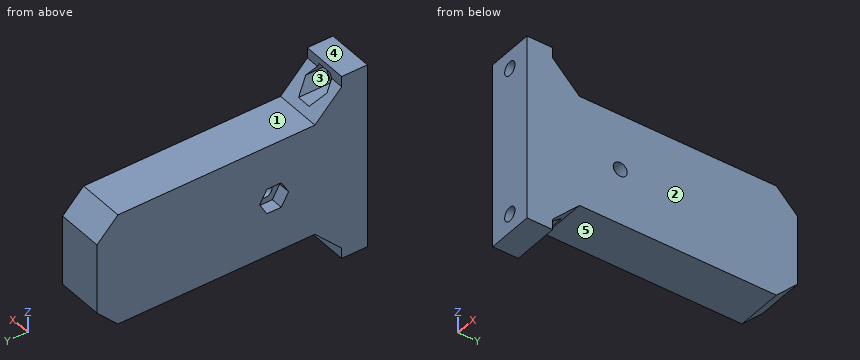
Autodesk Inventor part; units mm, degrees
ref_plane "YZ Plane" through (0, 0, 0) normal (1, 0, 0) x (0, 1, 0)
ref_plane "XZ Plane" through (0, 0, 0) normal (0, 1, 0) x (-1, 0, 0)
ref_plane "XY Plane" through (0, 0, 0) normal (0, 0, 1) x (1, 0, 0)
sketch "Эскиз1" plane through (0, 0, 0) normal (0, 1, 0) x (-1, 0, 0)
  line L0 (-5, 20) -> (5, 20)
  line L1 (5, 20) -> (5, -20)
  line L2 (5, -20) -> (-5, -20)
  line L3 (-5, -20) -> (-5, 20)
  line L4 (-5, 20) -> (5, -20) construction
  line L5 (5, 20) -> (-5, -20) construction
  point P0 (0, 0)
  dimension "d0" = 10
  dimension "d1" = 40
extrude "Выдавливание1" add sketch "Эскиз1" along normal blind 3
sketch "Эскиз2" plane through (0, 3, 0) normal (0, 1, 0) x (1, 0, 0)
  line L0 (-5, 20) -> (-5, -20)
  line L1 (5, -12) -> (-5, -12)
  line L2 (-5, -12) -> (-5, 12)
  line L3 (-5, 12) -> (5, 12)
  line L4 (5, 12) -> (5, -12)
  line L5 (5, -12) -> (-5, 12) construction
  line L6 (-5, -12) -> (5, 12) construction
  point P0 (0, 0)
  dimension "d4" = 24
extrude "Выдавливание2" add sketch "Эскиз2" along normal blind 55
sketch "Эскиз3" plane through (0, 3, 0) normal (0, 1, 0) x (1, 0, 0)
  circle A0 centre (0, -16) radius 1.5
  line L0 (-5, -12) -> (-5, -20)
  line L1 (-5, -20) -> (5, -20)
  point P0 (0, 0)
  dimension "d7" = 3
  dimension "d8" = 5
  dimension "d9" = 4
extrude "Выдавливание3" cut sketch "Эскиз3" against normal blind 20
mirror "Зеркальное отражение1" about plane through (0, 0, 0) normal (0, 0, 1) of "Выдавливание3"
sketch "Эскиз4" plane through (0, 3, 0) normal (0, 1, 0) x (1, 0, 0)
  circle A0 centre (0, -16) radius 1.5
  line L0 (-3.1, -16) -> (-1.55, -13.3153)
  line L1 (-1.55, -13.3153) -> (1.55, -13.3153)
  line L2 (1.55, -13.3153) -> (3.1, -16)
  line L3 (3.1, -16) -> (1.55, -18.6847)
  line L4 (1.55, -18.6847) -> (-1.55, -18.6847)
  line L5 (-1.55, -18.6847) -> (-3.1, -16)
  line L6 (-5, -12) -> (5, -12)
  line L7 (5, -20) -> (-5, -20)
  line L8 (-5, -20) -> (-5, -12)
  line L9 (-5, -12) -> (5, -12)
  line L10 (5, -12) -> (5, -20)
  line L11 (5, -20) -> (-5, -12) construction
  line L12 (-5, -20) -> (5, -12) construction
  point P0 (0, 0)
  dimension "d12" = 6.2
extrude "Выдавливание4" add sketch "Эскиз4" along normal blind 2.5 contours L6 L10 L7 L8
mirror "Зеркальное отражение2" about plane through (0, 0, 0) normal (0, 0, 1) of "Выдавливание4"
sketch "Эскиз5" plane through (5, 0, 20) normal (1, 0, 0) x (0, 0, -1)
  circle A0 centre (20, 20) radius 1.5
  line L0 (40, 0) -> (0, 0)
  point P0 (20, 0)
  dimension "d16" = 3
  dimension "d29" = 20
extrude "Выдавливание5" cut sketch "Эскиз5" against normal blind 27.5
sketch "Эскиз6" plane through (-5, 0, -20) normal (-1, 0, 0) x (0, 0, 1)
  circle A0 centre (20, 20) radius 1.5
  line L0 (20, 23.1) -> (22.6847, 21.55)
  line L1 (22.6847, 21.55) -> (22.6847, 18.45)
  line L2 (22.6847, 18.45) -> (20, 16.9)
  line L3 (20, 16.9) -> (17.3153, 18.45)
  line L4 (17.3153, 18.45) -> (17.3153, 21.55)
  line L5 (17.3153, 21.55) -> (20, 23.1)
  point P0 (20, 0)
  point P1 (0, 0)
  dimension "d20" = 6.2
extrude "Выдавливание6" cut sketch "Эскиз6" against normal blind 2.6
chamfer "Фаска1" distance 4.5 angle 45 2 edges at (0, 58, 12) (0, 58, -12)
chamfer "Фаска2" distance 5.75 angle 45 2 edges at (0, 5.5, 12) (0, 5.5, -12)
sketch "Эскиз7" plane through (0, 0, 0) normal (0, -1, 0) x (1, 0, 0)
  circle A0 centre (0, -16) radius 1.5
  circle A1 centre (0, 16) radius 1.5
  line L0 (5, 20) -> (-5, 20)
  line L1 (-5, 20) -> (-5, -20)
  line L2 (-5, -20) -> (5, -20)
  line L3 (5, -20) -> (5, 20)
  point P0 (0, 0)
properties part number "000.209 - Крепеж крышки"
Read the model definition and answer for the solid it produces. Units are mm, in the model's axes. Face numbers are marked on the shaded views. A direction names the side the tool comes from. Give positions to 0.01 mm unless a question says otherwise; leave off trailing zeros. Write each loop counter-clockwise with the first axis right and the second up, starting at its lowest first coordinate (ties: lowest second). Pieces come first, ordered by that corner, then holes. Notation, with made-up numbers: (-39.75, 25.5) -> (-21.75, 25.5) arc R20 cw to (-21.75, 30.5) -> close; hole circle Ø8 at (-40, 7). An arc over 180 degrees is marked (long way). Answer in a Markdown table with one row per item.
1) Each of these flat-tipped pins is pushed along its axis until it touches: pin 1 Ø3 at (x, y) = (-3.5, 20) entering from -Z; pin 2 Ø1 at (x, y) = (0, 21) entering from +Z; pin 3 Ø3.5 at (x, z) = (0, 16) entering from +Y. Where does it stop, or does it pass through?
Results list:
| item | result |
|---|---|
| pin 1 | z = -12 |
| pin 2 | z = 12 |
| pin 3 | y = 3 |
2) Section C-C on z = 10 is taken. Give the vertices of the cut face in (x, y), plus the area to 3 significant figures.
Results list:
| item | result |
|---|---|
| outline | (-5, 0) -> (5, 0) -> (5, 55.5) -> (-5, 55.5) -> close |
| area | 555 mm^2 |
3) Determine the mould class of the marked faces 1, 2 and 3 for opening direction Z: released by +Z, released by -Z, zero draft, split by the parting line, or undercut.
Results list:
| item | result |
|---|---|
| face 1 | released by +Z |
| face 2 | zero draft |
| face 3 | undercut |
4) Section A-A on y = 20 is taken. Give the vertices of the cut face in (x, z).
Results list:
| item | result |
|---|---|
| outline | (-5, -12) -> (5, -12) -> (5, -1.5) -> (-2.4, -1.5) -> (-2.4, -2.68) -> (-5, -2.68) -> close; (-5, 2.68) -> (-2.4, 2.68) -> (-2.4, 1.5) -> (5, 1.5) -> (5, 12) -> (-5, 12) -> close |
5) Section B-B on x = 0.5 is taken. Give the vertices of the cut face in (y, z).
Results list:
| item | result |
|---|---|
| outline | (0, -20) -> (5.5, -20) -> (5.5, -18.68) -> (3, -18.68) -> (3, -17.41) -> (0, -17.41) -> close; (0, -14.59) -> (3, -14.59) -> (3, -13.32) -> (9.93, -13.32) -> (11.25, -12) -> (53.5, -12) -> (58, -7.5) -> (58, 7.5) -> (53.5, 12) -> (11.25, 12) -> (9.93, 13.32) -> (3, 13.32) -> (3, 14.59) -> (0, 14.59) -> close; (0, 17.41) -> (3, 17.41) -> (3, 18.68) -> (5.5, 18.68) -> (5.5, 20) -> (0, 20) -> close; hole circle Ø3 at (20, 0) |
6) Section D-D on y = 44.5 is taken. Give the vertices of the cut face in (x, z).
Results list:
| item | result |
|---|---|
| outline | (-5, -12) -> (5, -12) -> (5, 12) -> (-5, 12) -> close |
7) Straight lines are drawn through the part: line 1 (Z direction, x = -1, y = 5); line 2 (Z direction, x = 0, y = 2.25); line 3 (X direction, y = 6, z = -16). For each, find the intervals that lie inside material, in ascending order. Write a range as [from, to].
Results list:
| item | result |
|---|---|
| line 1 | [-20, -18.68], [-13.32, 13.32], [18.68, 20] |
| line 2 | [-20, -17.5], [-14.5, 14.5], [17.5, 20] |
| line 3 | [-5, -3.1], [3.1, 5] |
8) A tool of negligible diameter and unlimited length cuts with its end or side. For the marked faces 4 and 5, from which of +Z, -Z, +X, -X, +Y, -Y can it reach the whole face along a straight path? Write none if from no direction.
Results list:
| item | result |
|---|---|
| face 4 | +Z, +X, -X, +Y, -Y |
| face 5 | -Z, +X, -X, +Y |
